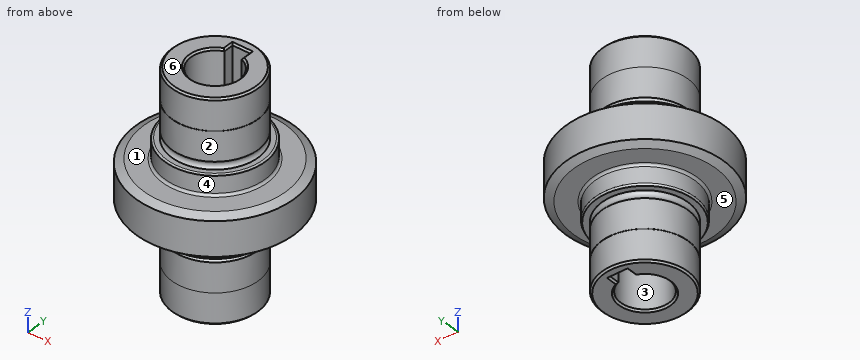
```python
from build123d import *

# Parameters (mm, degrees)
SKICA1_R                    = 22.9
P_IDAT_VYSUNUT_M1_DEPTH     = 31.5
SKICA2_R                    = 7
ODEBRAT_VYSUNUT_M1_DEPTH    = 71.836572475
SKICA3_W                    = 5
SKICA3_H                    = 4
ODEBRAT_VYSUNUT_M2_DEPTH    = 71.836572475
ODEBRAT_START               = -25.5
SKICA5_R                    = 22.9
SKICA5_R_2                  = 14.5
ODEBRAT_VYSUNUT_M4_DEPTH    = 25.5
ODEBRAT_START_2             = -19.7
SKICA6_R                    = 14.5
SKICA6_R_2                  = 12.5
ODEBRAT_VYSUNUT_M5_DEPTH    = 19.7
ODEBRAT_START_3             = -9
SKICA7_R                    = 12.5
SKICA7_R_2                  = 12.45
ODEBRAT_VYSUNUT_M6_DEPTH    = 9
ZKOSEN_4_SIZE               = 0.6
ZKOSEN_4_SIZE2              = 0.279784595
ZKOSEN_4_OF_ZRCADLIT2_SIZE2 = 0.6
ZKOSEN_4_OF_ZRCADLIT2_SIZE  = 0.279784595
ZKOSEN_1_SIZE               = 0.5
ZAOBLIT1_R                  = 0.65
ZKOSEN_2_SIZE               = 1
ZKOSEN_2_SIZE2              = 2.299842547
ZKOSEN_3_SIZE               = 2.3
ZKOSEN_3_SIZE2              = 1.072507614


with BuildPart() as part:
    # Skica1 → Přidat vysunutím1 (new, symmetric)
    with BuildSketch(Plane.XY):
        Circle(SKICA1_R)
    extrude(amount=P_IDAT_VYSUNUT_M1_DEPTH, both=True)

    # Skica2 → Odebrat vysunutím1 (cut, through all)
    with BuildSketch(Plane.XY.offset(31.5)):
        Circle(SKICA2_R)
    extrude(amount=-ODEBRAT_VYSUNUT_M1_DEPTH, mode=Mode.SUBTRACT)

    # Skica3 → Odebrat vysunutím2 (cut, through all)
    with BuildSketch(Plane.XY.offset(31.5)):
        with Locations((0, 7.5)):
            Rectangle(SKICA3_W, SKICA3_H)
    extrude(amount=-ODEBRAT_VYSUNUT_M2_DEPTH, mode=Mode.SUBTRACT)

    # Skica5 → Odebrat vysunutím4 (cut)
    with BuildSketch(Plane(origin=(0, 0, -31.5), x_dir=(-1, 0, 0), z_dir=(0, 0, -1)).offset(ODEBRAT_START)):
        Circle(SKICA5_R)
        Circle(SKICA5_R_2, mode=Mode.SUBTRACT)
    odebrat_vysunut_m4 = extrude(amount=ODEBRAT_VYSUNUT_M4_DEPTH, mode=Mode.SUBTRACT)

    # Skica6 → Odebrat vysunutím5 (cut)
    with BuildSketch(Plane(origin=(0, 0, -31.5), x_dir=(-1, 0, 0), z_dir=(0, 0, -1)).offset(ODEBRAT_START_2)):
        Circle(SKICA6_R)
        Circle(SKICA6_R_2, mode=Mode.SUBTRACT)
    odebrat_vysunut_m5 = extrude(amount=ODEBRAT_VYSUNUT_M5_DEPTH, mode=Mode.SUBTRACT)

    # Skica7 → Odebrat vysunutím6 (cut)
    with BuildSketch(Plane(origin=(0, 0, -31.5), x_dir=(-1, 0, 0), z_dir=(0, 0, -1)).offset(ODEBRAT_START_3)):
        Circle(SKICA7_R)
        Circle(SKICA7_R_2, mode=Mode.SUBTRACT)
    odebrat_vysunut_m6 = extrude(amount=ODEBRAT_VYSUNUT_M6_DEPTH, mode=Mode.SUBTRACT)

    # Zkosení4
    zkosen_4_edges = [part.edges().sort_by_distance(p)[0] for p in [
        (14.5, 0, -11.8),
    ]]
    zkosen_4_side = [part.faces().sort_by_distance(p)[0] for p in [
        (14.5, 0, -8.9),
    ]]
    chamfer(zkosen_4_edges, length=ZKOSEN_4_SIZE, length2=ZKOSEN_4_SIZE2, reference=zkosen_4_side[0])

    # Skica8 → Odebrat rotací1 (revolve, cut)
    with BuildSketch(Plane(origin=(0, 0, 0), x_dir=(0, 0, -1), z_dir=(1, 0, 0)), mode=Mode.PRIVATE) as odebrat_rotac_1_sk:
        with BuildLine():
            Line((11.8, -12.5), (14, -12.5))
            ThreePointArc((14, -12.5), (12.9, -11.892820323), (11.8, -12.5))
        make_face()
    odebrat_rotac_1 = revolve(odebrat_rotac_1_sk.sketch.rotate(Axis((0, 0, 0), (0, 0, -1)), 90), axis=Axis((0, 0, 0), (0, 0, -1)), mode=Mode.SUBTRACT)

    # Zrcadlit2: Odebrat vysunutím4, Odebrat vysunutím5, Odebrat vysunutím6, Odebrat rotací1 across plane
    add(odebrat_vysunut_m4.mirror(Plane.XY), mode=Mode.SUBTRACT)
    add(odebrat_vysunut_m5.mirror(Plane.XY), mode=Mode.SUBTRACT)
    add(odebrat_vysunut_m6.mirror(Plane.XY), mode=Mode.SUBTRACT)
    add(odebrat_rotac_1.mirror(Plane.XY), mode=Mode.SUBTRACT)

    # Zkosení4 of Zrcadlit2
    zkosen_4_of_zrcadlit2_edges = [part.edges().sort_by_distance(p)[0] for p in [
        (14.5, 0, 11.8),
    ]]
    chamfer(zkosen_4_of_zrcadlit2_edges, length=ZKOSEN_4_OF_ZRCADLIT2_SIZE, length2=ZKOSEN_4_OF_ZRCADLIT2_SIZE2)

    # Zkosení1
    zkosen_1_edges = [part.edges().sort_by_distance(p)[0] for p in [
        (0, -7, -31.5),
        (0, -7, 31.5),
        (2.5, 8.019174208, -31.5),
        (-2.5, 8.019174208, -31.5),
        (-2.5, 8.019174208, 31.5),
        (2.5, 8.019174208, 31.5),
        (0, 9.5, 31.5),
        (0, 9.5, -31.5),
        (12.45, 0, -31.5),
        (12.45, 0, 31.5),
    ]]
    chamfer(zkosen_1_edges, length=ZKOSEN_1_SIZE)

    # Zaoblit1
    zaoblit1_edges = [part.edges().sort_by_distance(p)[0] for p in [
        (14.5, 0, -6),
        (14.5, 0, 6),
    ]]
    fillet(zaoblit1_edges, radius=ZAOBLIT1_R)

    # Zkosení2
    zkosen_2_edges = [part.edges().sort_by_distance(p)[0] for p in [
        (-22.9, 0, -6),
    ]]
    zkosen_2_side = [part.faces().sort_by_distance(p)[0] for p in [
        (-22.9, 0, 0),
    ]]
    chamfer(zkosen_2_edges, length=ZKOSEN_2_SIZE, length2=ZKOSEN_2_SIZE2, reference=zkosen_2_side[0])

    # Zkosení3
    zkosen_3_edges = [part.edges().sort_by_distance(p)[0] for p in [
        (-22.9, 0, 6),
    ]]
    zkosen_3_side = [part.faces().sort_by_distance(p)[0] for p in [
        (15.797709812, 0, 6),
    ]]
    chamfer(zkosen_3_edges, length=ZKOSEN_3_SIZE, length2=ZKOSEN_3_SIZE2, reference=zkosen_3_side[0])


solid = part.part
```
The model under review builds one solid part; all positions refer to its coordinate system, in mm. Face numbers are marked on the shaded views. A direction names the side the tool comes from. Coordinates: 2 decimals unless noted, no trailing zeros. Loops run counter-clockwise (first coordinate to the right, second up) from the corner with the lowest first, then second, coordinate; pieces in that order, holes last. Notation, with made-up numbers: (5, 11) -> (13, 11) arc R5 cw to (13, 17) -> close; hole circle Ø1 at (54.5, 47.5). An arc over 180 degrees is marked (long way). Answer as CSV lines item,"result".
Item 1: Insertion check: pin 1 (2 mm diameter, centred on y = 9, z = 13.5, fed in from -X); pin 2 (12 mm diameter, centred on y = 8.5, z = 17, fed in from -X); pin 3 (1.5 mm diameter, centred on x = 0, z = 2, fed in from -Y); pin 4 (2 mm diameter, centred on y = -14.5, z = -18.5, fed in from -X). Each pin has a flat end and moves straight along its axis. Give the tip position at first contact, or say it passes through.
Results below:
pin 1,"stops at x = -9.49"
pin 2,"stops at x = -13.17"
pin 3,"stops at y = -22.9"
pin 4,"passes through"
Item 2: Take a section at A-A, the plane z = -26. State the section outline as (x, y) points, and give its area (3 significant figures).
Results below:
outline,"circle Ø24.9 at (0, 0); hole (-2.5, 6.54) arc R7 ccw (long way) to (2.5, 6.54) -> (2.5, 9.5) -> (-2.5, 9.5) -> close"
area,"320 mm2"
Item 3: Take a section at B-B, the plane z = 8. State the section outline as (x, y) points.
Results below:
outline,"circle Ø29 at (0, 0); hole (-2.5, 6.54) arc R7 ccw (long way) to (2.5, 6.54) -> (2.5, 9.5) -> (-2.5, 9.5) -> close"
Item 4: Draft analysis for pull direction Y (two halves, no side actions). For the marked faces 1, 2 and 3, state which applies: +Y half, -Y half, draft (parallel to the pull), parting line (faces both ways), or undercut.
Results below:
face 1,"draft"
face 2,"parting line"
face 3,"undercut"
Item 5: For L1, parallel to Y at x = 0, z = 24; L2, parallel to X at y = 0, z = -4; L3, parallel to Y at x = 0, z = 14, list the stretches that pass through material, from the lowest coordinate up.
Results below:
L1,"y = -12.45 to -7, 9.5 to 12.45"
L2,"x = -22.9 to -7, 7 to 22.9"
L3,"y = -12.5 to -7, 9.5 to 12.5"
Item 6: Machinability: for the marked faces 4, 5 and 6, which of the approach directions +Z, -Z, +X, -X, +Y, -Y give a long, thin tool a straight path to every point of the face, cutting with its end or side? Answer none if there is none.
Results below:
face 4,"+Z"
face 5,"-Z"
face 6,"+Z, +X, -X, +Y, -Y"
